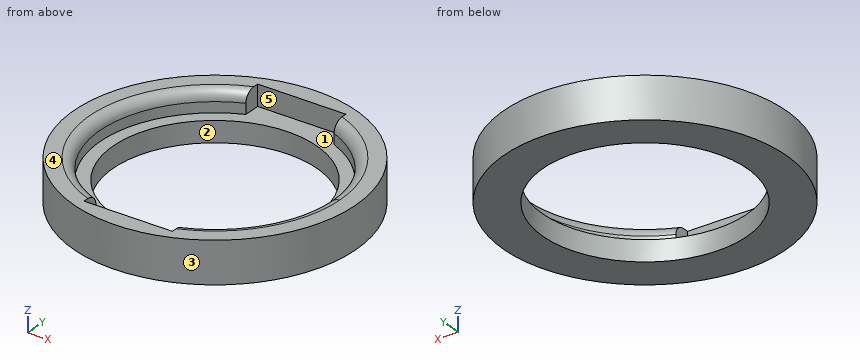
```python
from build123d import *

# Parameters (mm, degrees)
F0_R     = 13.5
F1_DEPTH = 4
F2_R     = 13.5
F2_R_2   = 9.75
F3_DEPTH = 2
F4_R     = 1


with BuildPart() as f1:
    # F0 (on Top) → F1 (new body)
    with BuildSketch(Plane.XY):
        Circle(F0_R)
        with BuildLine():
            ThreePointArc((4.25, 10.1458119439), (9.158329542, 6.0930288035), (11, 0))
            ThreePointArc((11, 0), (9.158329542, -6.0930288035), (4.25, -10.1458119439))
            Line((4.25, -10.1458119439), (4.25, -11.75))
            Line((4.25, -11.75), (-4.25, -11.75))
            Line((-4.25, -11.75), (-4.25, -10.1458119439))
            ThreePointArc((-4.25, -10.1458119439), (-11, 0), (-4.25, 10.1458119439))
            Line((-4.25, 10.1458119439), (-4.25, 11.75))
            Line((-4.25, 11.75), (4.25, 11.75))
            Line((4.25, 11.75), (4.25, 10.1458119439))
        make_face(mode=Mode.SUBTRACT)
    extrude(amount=F1_DEPTH)

    # F2 (on Top) → F3 (join)
    with BuildSketch(Plane.XY):
        Circle(F2_R)
        Circle(F2_R_2, mode=Mode.SUBTRACT)
    extrude(amount=F3_DEPTH)

    # F4
    f4_edges = [f1.edges().sort_by_distance(p)[0] for p in [
        (11, 0, 4),
        (-11, 0, 4),
    ]]
    fillet(f4_edges, radius=F4_R)


solid = f1.part
```
Part model, mm, in its own coordinate system. Face numbers are marked on the shaded views. A direction names the side the tool comes from. Round coordinates to 2 decimals unless told otherwise and drop trailing zeros. Loops run counter-clockwise (first coordinate to the right, second up) from the corner with the lowest first, then second, coordinate; pieces in that order, holes last.
1. Drill centre lines: line 1 along Y through (x, z) = (0, 0.95); line 2 along X through (y, z) = (-4.75, 1.05); line 3 along Y through (x, z) = (1.5, 3.8). Where is each one in solid material? Low to high.
Solutions:
line 1: y = -13.5 to -9.75, 9.75 to 13.5
line 2: x = -12.64 to -8.51, 8.51 to 12.64
line 3: y = -13.42 to -11.75, 11.75 to 13.42
2. Two-plate mould, pull along Y, no slides. Class the marked faces 3, 4 and 5: pulls with the +Y half, pulls with the -Y half, needs draft (parallel to the pull), parting line crosses it, or undercut.
Solutions:
face 3: parting line crosses it
face 4: needs draft
face 5: undercut
3. Flat gauge pins, fed straight in: pin 1 (0.5 mm diameter, centred on y = -10.5, z = 3.5, fed in from +X); pin 2 (0.8 mm diameter, centred on y = 11, z = 3, fed in from +X); pin 3 (1.5 mm diameter, centred on y = 4, z = 3, fed in from +X); pin 4 (6 mm diameter, centred on x = -5.5, y = 9, fed in from +Z). Where does each tip first touch, or does it go through?
Solutions:
pin 1: stops at x = 8.79
pin 2: stops at x = 8.36
pin 3: stops at x = 13.1
pin 4: stops at z = 4
4. Slice it at B-B (z = 1.65). Give the cut face in (x, y).
Solutions:
outline: circle Ø27 at (0, 0); hole circle Ø19.5 at (0, 0)
5. Slice it at A-A (x = 0). Give the cut face in (y, z).
Solutions:
outline: (-13.5, 0) - (-9.75, 0) - (-9.75, 2) - (-11.75, 2) - (-11.75, 4) - (-13.5, 4) - close; (9.75, 0) - (13.5, 0) - (13.5, 4) - (11.75, 4) - (11.75, 2) - (9.75, 2) - close
6. 3-axis set-ups, long thin cutter, end or side, ignore diameter. For the marked faces 1 and 2: which of +Z, -Z, +X, -X, +Y, -Y reach the whole face in a straight line?
Solutions:
face 1: +Z
face 2: +Z, -Z
